```python
from build123d import *

# Parameters (mm, degrees)
F1_DEPTH = 609.6
F2_W     = 25.4
F2_H     = 101.6
F2_H_2   = 114.3
F3_DEPTH = 609.6
F4_W     = 152.4
F4_H     = 25.4
F4_W_2   = 25.4
F5_DEPTH = 1016
F7_DEPTH = 25.4
F8_DEPTH = 25.4


with BuildPart() as f1:
    # F0 (on Top) → F1 (new body)
    with BuildSketch(Plane.XY):
        Polygon((304.8, 838.2), (0, 838.2), (0, 419.1), (0, 0), (304.8, 0), (304.8, 25.4), (25.4, 25.4), (25.4, 203.2), (304.8, 203.2), (304.8, 215.9), (304.8, 228.6), (25.4, 228.6), (25.4, 406.4), (304.8, 406.4), (304.8, 419.1), (304.8, 431.8), (25.4, 431.8), (25.4, 609.6), (304.8, 609.6), (304.8, 622.3), (304.8, 635), (25.4, 635), (25.4, 812.8), (304.8, 812.8), align=None)
    extrude(amount=-F1_DEPTH)

    # F2 (on face) → F3 (join)
    with BuildSketch(Plane.XY):
        with Locations((292.1, 889)):
            Rectangle(F2_W, F2_H)
        with Locations((12.7, 895.35)):
            Rectangle(F2_W, F2_H_2)
        with Locations((12.7, -57.15)):
            Rectangle(F2_W, F2_H_2)
        with Locations((292.1, -50.8)):
            Rectangle(F2_W, F2_H)
    extrude(amount=-F3_DEPTH)

    # F4 (on Front) → F5 (cut, symmetric)
    with BuildSketch(Plane.XZ):
        with Locations((101.6, -12.7)):
            Rectangle(F4_W, F4_H)
        with Locations((292.1, -12.7)):
            Rectangle(F4_W_2, F4_H)
        with Locations((101.6, -596.9)):
            Rectangle(F4_W, F4_H)
        with Locations((292.1, -596.9)):
            Rectangle(F4_W_2, F4_H)
    extrude(amount=F5_DEPTH, both=True, mode=Mode.SUBTRACT)

    # F6 (on face) → F7 (cut, through all)
    with BuildSketch(Plane.YZ.offset(304.8)):
        Polygon((-101.6, -254), (-101.6, -304.8), (-101.6, -355.6), (-50.8, -355.6), (-50.8, -304.8), (-50.8, -254), align=None)
        Polygon((-50.8, -127), (-50.8, -76.2), (-101.6, -76.2), (-101.6, -127), (-101.6, -177.8), (-50.8, -177.8), align=None)
        Polygon((-101.6, -533.4), (-50.8, -533.4), (-50.8, -482.6), (-50.8, -431.8), (-101.6, -431.8), (-101.6, -482.6), align=None)
        Polygon((889.8554785728, -355.6), (940.6554785728, -355.6), (940.6554785728, -304.8), (940.6554785728, -254), (889.8554785728, -254), (889.8554785728, -304.8), align=None)
        Polygon((940.6554785728, -533.4), (940.6554785728, -482.6), (940.6554785728, -431.8), (889.8554785728, -431.8), (889.8554785728, -482.6), (889.8554785728, -533.4), align=None)
        Polygon((889.8554785728, -177.8), (940.6554785728, -177.8), (940.6554785728, -127), (940.6554785728, -76.2), (889.8554785728, -76.2), (889.8554785728, -127), align=None)
    extrude(amount=-F7_DEPTH, mode=Mode.SUBTRACT)

    # F6 (on face) → F8 (cut)
    with BuildSketch(Plane.YZ.offset(304.8)):
        Polygon((-101.6, -254), (-101.6, -304.8), (-101.6, -355.6), (-50.8, -355.6), (-50.8, -304.8), (-50.8, -254), align=None)
        Polygon((-50.8, -127), (-50.8, -76.2), (-101.6, -76.2), (-101.6, -127), (-101.6, -177.8), (-50.8, -177.8), align=None)
        Polygon((-101.6, -533.4), (-50.8, -533.4), (-50.8, -482.6), (-50.8, -431.8), (-101.6, -431.8), (-101.6, -482.6), align=None)
        Polygon((889.8554785728, -355.6), (940.6554785728, -355.6), (940.6554785728, -304.8), (940.6554785728, -254), (889.8554785728, -254), (889.8554785728, -304.8), align=None)
        Polygon((940.6554785728, -533.4), (940.6554785728, -482.6), (940.6554785728, -431.8), (889.8554785728, -431.8), (889.8554785728, -482.6), (889.8554785728, -533.4), align=None)
        Polygon((889.8554785728, -177.8), (940.6554785728, -177.8), (940.6554785728, -127), (940.6554785728, -76.2), (889.8554785728, -76.2), (889.8554785728, -127), align=None)
    extrude(amount=-F8_DEPTH, mode=Mode.SUBTRACT)


solid = f1.part
```
Design review of the part built by this model. Coordinates are the model's own, in mm. A direction names the side the tool comes from. Coordinates: 2 decimals unless noted, no trailing zeros. Write each loop counter-clockwise with the first axis right and the second up, starting at its lowest first coordinate (ties: lowest second). Pieces come first, ordered by that corner, then holes. Notation, with made-up numbers: M 29,49.5 L 81,49.5 A26 cw 81,78.5 Z; hole C -17,4.25 d2. An arc over 180 degrees is marked long. Answer as a JSON object with one key per item and string values.
Item 1: Draft analysis for pull direction Z (two halves, no side actions). For faces 6 (the flat face through (292, 915, -431.8)), 7 (the flat face through (292, 622, -584.2)), 8 (the flat face through (292, -50.8, -483)), 9 (the flat face through (177.8, 13, -597)), state which applies: pulls with the +Z half, pulls with the -Z half, needs draft (parallel to the pull), parting line crosses it, or undercut.
Outcome:
{"face 6": "undercut", "face 7": "pulls with the -Z half", "face 8": "undercut", "face 9": "needs draft"}
Item 2: Add section C-C, the plane x = 189. Give the boundary of the cut face in (y, z), and give its area (3 significant figures).
Outcome:
{"outline": "M 0,-609.6 L 25.4,-609.6 L 25.4,0 L 0,0 Z; M 203.2,-609.6 L 228.6,-609.6 L 228.6,0 L 203.2,0 Z; M 406.4,-609.6 L 431.8,-609.6 L 431.8,0 L 406.4,0 Z; M 609.6,-609.6 L 635,-609.6 L 635,0 L 609.6,0 Z; M 812.8,-609.6 L 838.2,-609.6 L 838.2,0 L 812.8,0 Z", "area": "77,400 mm²"}
Item 3: Wall thickness on probe 1 along Y at (x, z) = (77.5, -31); probe 2 along X at (y, z) = (861, -574); probe 3 along X at (y, z) = (-65, -513): over which ranges is each line inside the solid? List them lowest first.
Outcome:
{"probe 1": "0 to 25.4, 203.2 to 228.6, 406.4 to 431.8, 609.6 to 635, 812.8 to 838.2", "probe 2": "0 to 25.4, 279.4 to 304.8", "probe 3": "0 to 25.4"}
Item 4: Machinability: for faces 1 (the flat face through (101, 13, -25.4)), 2 (the flat face through (101, 13, -584.2)), 3 (the flat face through (292, 419, -25.4)), 4 (the flat face through (163, 406.4, -301)), 5 (the flat face through (279.4, 13, -597)), which of the approach directions +Z, -Z, +X, -X, +Y, -Y give a long, thin tool a straight path to every point of the face, cutting with its end or side? Answer none if there is none.
Outcome:
{"face 1": "+Z, +Y, -Y", "face 2": "-Z, +Y, -Y", "face 3": "+Z, +X, +Y, -Y", "face 4": "+Z, -Z, +X", "face 5": "-Z, +X, +Y, -Y"}
Item 5: Add section A-A, the plane x = 51. Give the boundary of the cut face in (y, z), and give its area (3 significant figures).
Outcome:
{"outline": "M 0,-584.2 L 25.4,-584.2 L 25.4,-25.4 L 0,-25.4 Z; M 203.2,-584.2 L 228.6,-584.2 L 228.6,-25.4 L 203.2,-25.4 Z; M 406.4,-584.2 L 431.8,-584.2 L 431.8,-25.4 L 406.4,-25.4 Z; M 609.6,-584.2 L 635,-584.2 L 635,-25.4 L 609.6,-25.4 Z; M 812.8,-584.2 L 838.2,-584.2 L 838.2,-25.4 L 812.8,-25.4 Z", "area": "71,000 mm²"}
Item 6: Add section D-D, the plane y = 462.5. Give the boundary of the cut face in (x, z), and give its area (3 significant figures).
Outcome:
{"outline": "M 0,-609.6 L 25.4,-609.6 L 25.4,0 L 0,0 Z", "area": "15,500 mm²"}
Item 7: Add section B-B, the plane z = -49.5. Give the boundary of the cut face in (x, y).
Outcome:
{"outline": "M 0,-114.3 L 25.4,-114.3 L 25.4,0 L 279.4,0 L 279.4,-101.6 L 304.8,-101.6 L 304.8,25.4 L 25.4,25.4 L 25.4,203.2 L 304.8,203.2 L 304.8,228.6 L 25.4,228.6 L 25.4,406.4 L 304.8,406.4 L 304.8,431.8 L 25.4,431.8 L 25.4,609.6 L 304.8,609.6 L 304.8,635 L 25.4,635 L 25.4,812.8 L 304.8,812.8 L 304.8,939.8 L 279.4,939.8 L 279.4,838.2 L 25.4,838.2 L 25.4,952.5 L 0,952.5 Z"}
Item 8: Insertion check: pin 1 Ø20.5 at (x, y) = (294, 617.5) entering from +Z; pin 2 Ø20.5 at (x, y) = (290, -84.5) entering from -Z; pin 3 Ø1.5 at (x, z) = (67, -96.5) entering from +Y. Each pin has a flat end and moves straight along its axis. Give the tip position at first contact, or say it passes through.
Outcome:
{"pin 1": "z = -25.4", "pin 2": "z = -584.2", "pin 3": "y = 838.2"}
